Answer from the drawing. Dimensions are ordinates in mm from the lowest x, y and z of the part. A direction names the side the tool comes from. Coordinates: 2 decimals unless noted, no trailing zeros. Write each loop counter-clockwise with the first axis right and the second up, starting at its lowest first coordinate (ties: lowest second). Pieces come first, ordered by that corner, then holes. Notation, with made-up numbers: M 67.5,19 L 114.5,19 A16 ccw 114.5,28 Z; hole C -29.75,-12.5 d10. An arc over 180 degrees is marked long. Put each result on its own line as item: value. Start each with the question number.
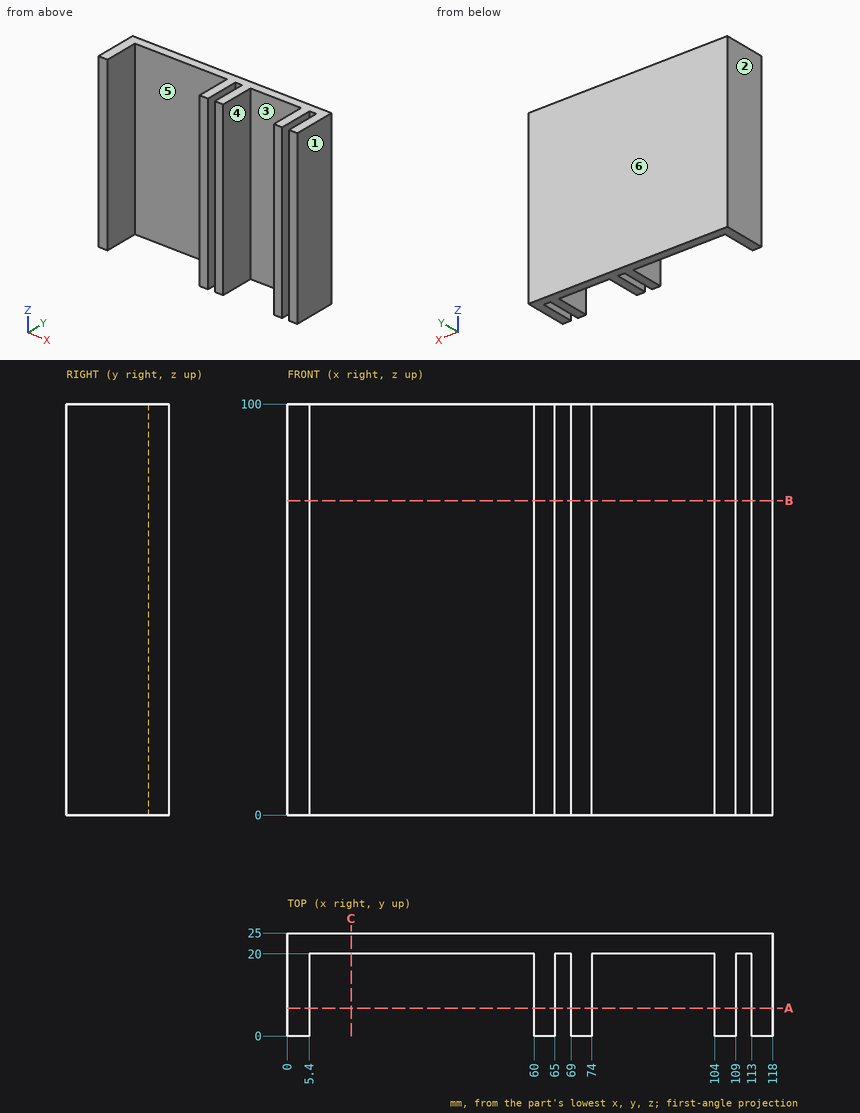
1) For the marked faces 5 and 6, determine the directions among +Z, -Z, +X, -X, +Y, -Y from which every point of the face is accessible in a straight line to the end or side of a thin tool.
2) Straight lines are drawn through the part: probe 1 along X at (y, z) = (13, 93.5); probe 2 along Y at (x, z) = (29.5, 17.5). For each, find the intervals that lie inside material, in ascending order.
3) Given pin 1 Ø15 at (x, z) = (87, 44) entering from -Y, flat-ended and moving along its own axis, determine where the tip first touches the part or whether it passes through.
4) Determine the mould class of the marked faces 1, 2, 3 and 4 for opening direction X: +X half, -X half, draft (parallel to the pull), parting line (faces both ways), or undercut.
5) A cutting plane is placed at B-B on z = 76.5. Write down the section's boundary in (x, y).
6) A cutting plane is placed at C-C on x = 15.5. Write down the section's boundary in (y, z).
7) A cutting plane is placed at A-A on y = 6.75. Write down the section's boundary in (x, z), then the cut area to 3 significant figures.
Answers follow:
1. face 5: +Z, -Z, -Y
1. face 6: +Z, -Z, +X, -X, +Y
2. probe 1: x = 0 to 5.4, 60 to 65, 69 to 74, 104 to 109, 113 to 118
2. probe 2: y = 20 to 25
3. pin 1: stops at y = 20
4. face 1: +X half
4. face 2: -X half
4. face 3: undercut
4. face 4: undercut
5. outline: M 0,0 L 5.4,0 L 5.4,20 L 60,20 L 60,0 L 65,0 L 65,20 L 69,20 L 69,0 L 74,0 L 74,20 L 104,20 L 104,0 L 109,0 L 109,20 L 113,20 L 113,0 L 118,0 L 118,25 L 0,25 Z
6. outline: M 20,0 L 25,0 L 25,100 L 20,100 Z
7. outline: M 0,0 L 5.4,0 L 5.4,100 L 0,100 Z; M 60,0 L 65,0 L 65,100 L 60,100 Z; M 69,0 L 74,0 L 74,100 L 69,100 Z; M 104,0 L 109,0 L 109,100 L 104,100 Z; M 113,0 L 118,0 L 118,100 L 113,100 Z
7. area: 2,540 mm²
